Verification items for this drawing (mm, ordinates from the low corner). Round coordinates to 2 decimals unless told otherwise and drop trailing zeros. Write each loop counter-clockwise with the first axis right and the second up, starting at its lowest first coordinate (ties: lowest second). Pieces come first, ordered by that corner, then holes. Notation, with made-up numbers: (-14.75, 27.5) -> (14.25, 27.5) arc R26 cw to (14.25, 50.5) -> close; hole circle Ø10 at (-35.75, 45). An arc over 180 degrees is marked (long way). One line per question, with ' | ' between items.
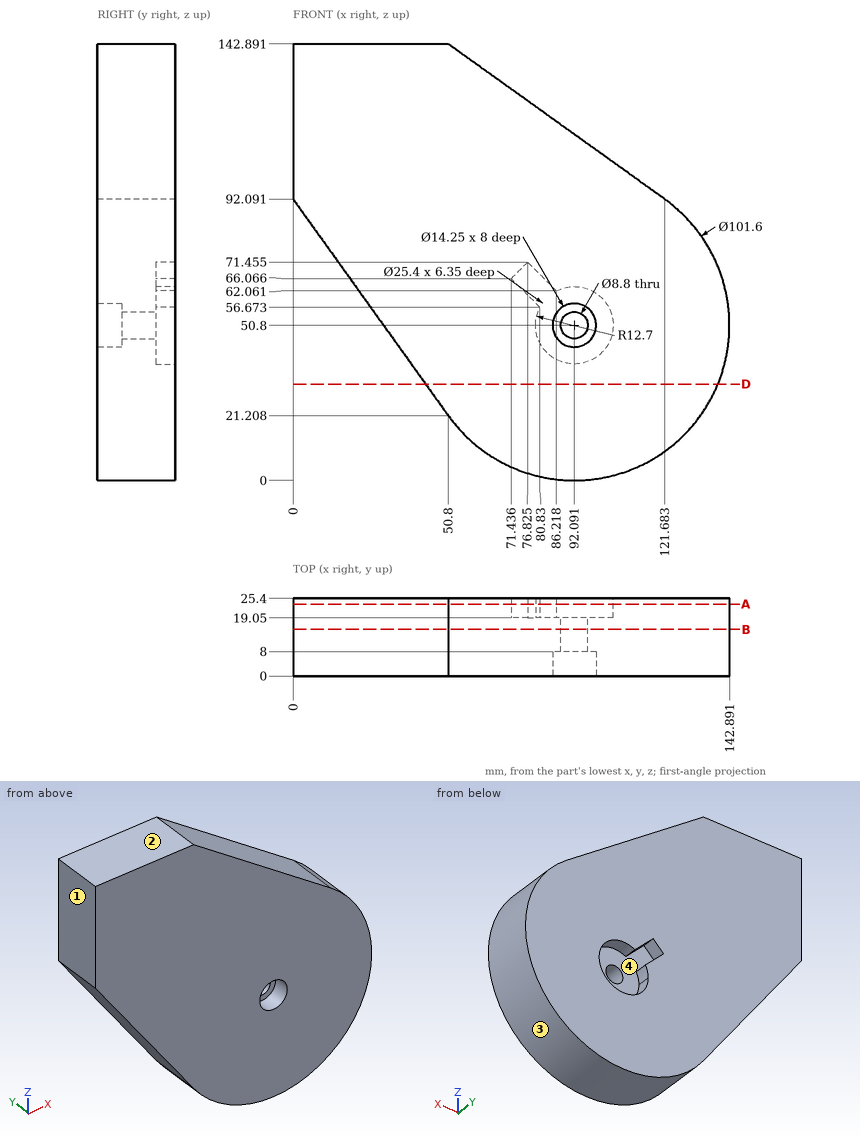
(1) Material ranges on line 1 (X direction, y = 15.25, z = 50.8); line 2 (Z direction, x = 97, y = 5.25) (1 decimal); line 3 (X direction, y = 3, z = 50.8) (1 decimal), recorded low to high.
Resolved:
line 1: x = 29.59 to 87.69, 96.49 to 142.89 | line 2: z = 0.2 to 45.6, 56 to 109.8 | line 3: x = 29.6 to 85, 99.2 to 142.9
(2) Go/stop test with flat-tipped pins: pin 1 (5 mm diameter, centred on y = 6, z = 39, fed in from -X); pin 2 (8 mm diameter, centred on x = 92.09, z = 50.8, fed in from -Y); pin 3 (4 mm diameter, centred on y = 3.5, z = 113.5, fed in from +X); pin 4 (1 mm diameter, centred on x = 92.5, y = 10, fed in from +Z) (1 decimal). Record where each tip stops, or that it passes through.
Resolved:
pin 1: stops at x = 36.26 | pin 2: passes through | pin 3: stops at x = 94.6 | pin 4: stops at z = 113.4
(3) Draft check along X on the marked faces 1, 2, 3 and 4. Enter one of: +X half, -X half, draft (parallel to the pull), parting line (faces both ways), or undercut.
Resolved:
face 1: -X half | face 2: draft | face 3: parting line | face 4: undercut
(4) Sectioned sample at A-A on y = 23.5. Record the cut outline in (x, z) (1 decimal), then the cut area to 3 significant figures.
Resolved:
outline: (0, 92.1) -> (50.8, 21.2) arc R50.8 ccw (long way) to (121.7, 92.1) -> (50.8, 142.9) -> (0, 142.9) -> close; hole (71.4, 66.1) -> (80.8, 56.7) arc R12.7 ccw (long way) to (86.2, 62.1) -> (76.8, 71.5) -> close | area: 13,000 mm2
(5) Sectioned sample at B-B on y = 15.25. Record the cut outline in (x, z).
Resolved:
outline: (0, 92.09) -> (50.8, 21.21) arc R50.8 ccw (long way) to (121.68, 92.09) -> (50.8, 142.89) -> (0, 142.89) -> close; hole circle Ø8.8 at (92.09, 50.8)
(6) Sectioned sample at D-D on z = 31.5. Record the cut outline in (x, y).
Resolved:
outline: (43.42, 0) -> (139.08, 0) -> (139.08, 25.4) -> (43.42, 25.4) -> close
